Verification items for the finished model (mm, model axes). Give positions to 0.01 mm unless a question says otherwise; leave off trailing zeros. Order: outer loops, then holes, each group sorted by start corner. A loop starts at its lowest first (then second) coordinate and runs counter-clockwise, first axis right, second up.
(1) Gauge pin test, flat ends, axial feed: pin 1 (0.9 mm diameter, centred on y = 1.5, z = 267.5, fed in from -X); pin 2 (0.9 mm diameter, centred on x = 262, y = 1.5, fed in from -Z); pin 3 (1.5 mm diameter, centred on x = 227, y = 2, fed in from -Z); pin 4 (5 mm diameter, centred on x = 214, z = 124.5, fed in from +Y). Record the tip position at first contact, or that the pin passes through.
(2) Scan lines: L1, parallel to Z at x = 187, y = 2.8; L2, parallel to X at y = 2.4, z = 94.5; L3, parallel to X at y = 0.2, z = 154. Record each from-to range of solid material in increasing order.
(3) Sectioned sample at C-C on z = 191. Record the cut outline in (x, y).
(4) Sectioned sample at A-A on y = 1.3. Record the cut outline in (x, z).
(5) Sectioned sample at D-D on x = 137.5. Record the cut outline in (y, z).
(6) Sectioned sample at B-B on x = 178.5. Record the cut outline in (y, z), plus the area to 3 significant figures.
Autodesk Inventor part; units mm, degrees
ref_plane "YZ Plane" through (0, 0, 0) normal (1, 0, 0) x (0, 1, 0)
ref_plane "XZ Plane" through (0, 0, 0) normal (0, 1, 0) x (-1, 0, 0)
ref_plane "XY Plane" through (0, 0, 0) normal (0, 0, 1) x (1, 0, 0)
sketch "Sketch1" plane through (0, 0, 0) normal (0, 1, 0) x (-1, 0, 0)
  circle A0 centre (0, 0) radius 250
  circle A1 centre (0, 0) radius 270
  line L0 (270, 0) -> (250, 0)
  line L1 (-270, 0) -> (-250, 0)
  line L2 (0, 0) -> (-250, 0) construction
  line L3 (0, 250) -> (0, 0) construction
  line L4 (0, 270) -> (0, 250)
  line L5 (-250, 0) -> (-270, 0)
  line L6 (-254, 7) -> (-266, 7)
  line L7 (-266, 7) -> (-263.4522, 0)
  line L8 (-254, 7) -> (-256.5478, 0)
  line L9 (-260, 0) -> (-260, 7) construction
  line L10 (-255.1125, 57.8859) -> (-246.8075, 86.7134)
  line L11 (-246.8075, 86.7134) -> (-243.7326, 85.8275)
  line L12 (-243.7326, 85.8275) -> (-252.0376, 57)
  line L13 (-252.0376, 57) -> (-255.1125, 57.8859)
  line L14 (-255.1125, 57.8859) -> (-243.7326, 85.8275) construction
  line L15 (-246.8075, 86.7134) -> (-252.0376, 57) construction
  circle A2 centre (0, 0) radius 260 construction
  line L16 (-7, -254) -> (0, -256.5478)
  line L17 (-7, -266) -> (0, -263.4522)
  line L18 (-7, -254) -> (-7, -266)
  line L19 (254, -7) -> (256.5478, 0)
  line L20 (266, -7) -> (263.4522, 0)
  line L21 (254, -7) -> (266, -7)
  line L22 (7, 254) -> (0, 256.5478)
  line L23 (7, 266) -> (0, 263.4522)
  line L24 (7, 254) -> (7, 266)
  line L25 (-249.8769, -77.4256) -> (-257.0983, -48.3078)
  line L26 (-246.771, -76.6553) -> (-249.8769, -77.4256)
  line L27 (-253.9924, -47.5375) -> (-246.771, -76.6553)
  line L28 (-257.0983, -48.3078) -> (-253.9924, -47.5375)
  line L29 (-177.6869, -191.991) -> (-198.4998, -170.3849)
  line L30 (-175.3822, -189.771) -> (-177.6869, -191.991)
  line L31 (-196.1951, -168.1649) -> (-175.3822, -189.771)
  line L32 (-198.4998, -170.3849) -> (-196.1951, -168.1649)
  line L33 (-57.8859, -255.1125) -> (-86.7134, -246.8075)
  line L34 (-57, -252.0376) -> (-57.8859, -255.1125)
  line L35 (-85.8275, -243.7326) -> (-57, -252.0376)
  line L36 (-86.7134, -246.8075) -> (-85.8275, -243.7326)
  line L37 (77.4256, -249.8769) -> (48.3078, -257.0983)
  line L38 (76.6553, -246.771) -> (77.4256, -249.8769)
  line L39 (47.5375, -253.9924) -> (76.6553, -246.771)
  line L40 (48.3078, -257.0983) -> (47.5375, -253.9924)
  line L41 (191.991, -177.6869) -> (170.3849, -198.4998)
  line L42 (189.771, -175.3822) -> (191.991, -177.6869)
  line L43 (168.1649, -196.1951) -> (189.771, -175.3822)
  line L44 (170.3849, -198.4998) -> (168.1649, -196.1951)
  line L45 (255.1125, -57.8859) -> (246.8075, -86.7134)
  line L46 (252.0376, -57) -> (255.1125, -57.8859)
  line L47 (243.7326, -85.8275) -> (252.0376, -57)
  line L48 (246.8075, -86.7134) -> (243.7326, -85.8275)
  line L49 (249.8769, 77.4256) -> (257.0983, 48.3078)
  line L50 (246.771, 76.6553) -> (249.8769, 77.4256)
  line L51 (253.9924, 47.5375) -> (246.771, 76.6553)
  line L52 (257.0983, 48.3078) -> (253.9924, 47.5375)
  line L53 (177.6869, 191.991) -> (198.4998, 170.3849)
  line L54 (175.3822, 189.771) -> (177.6869, 191.991)
  line L55 (196.1951, 168.1649) -> (175.3822, 189.771)
  line L56 (198.4998, 170.3849) -> (196.1951, 168.1649)
  line L57 (57.8859, 255.1125) -> (86.7134, 246.8075)
  line L58 (57, 252.0376) -> (57.8859, 255.1125)
  line L59 (85.8275, 243.7326) -> (57, 252.0376)
  line L60 (86.7134, 246.8075) -> (85.8275, 243.7326)
  line L61 (-77.4256, 249.8769) -> (-48.3078, 257.0983)
  line L62 (-76.6553, 246.771) -> (-77.4256, 249.8769)
  line L63 (-47.5375, 253.9924) -> (-76.6553, 246.771)
  line L64 (-48.3078, 257.0983) -> (-47.5375, 253.9924)
  line L65 (-191.991, 177.6869) -> (-170.3849, 198.4998)
  line L66 (-189.771, 175.3822) -> (-191.991, 177.6869)
  line L67 (-168.1649, 196.1951) -> (-189.771, 175.3822)
  line L68 (-170.3849, 198.4998) -> (-168.1649, 196.1951)
  point P0 (260, 0)
  point P1 (-260, 0)
  point P2 (-249.4226, 71.8567)
  point P3 (-49.7078, 255.2041)
  point P4 (-253.5751, 57.4429)
  point P5 (-245.2701, 86.2705)
  point P6 (-7, -260)
  point P7 (260, -7)
  point P8 (7, 260)
  point P9 (-248.3239, -77.0405)
  point P10 (-255.5453, -47.9226)
  point P11 (-176.5346, -190.881)
  point P12 (-197.3475, -169.2749)
  point P13 (-57.4429, -253.5751)
  point P14 (-86.2705, -245.2701)
  point P15 (77.0405, -248.3239)
  point P16 (47.9226, -255.5453)
  point P17 (190.881, -176.5346)
  point P18 (169.2749, -197.3475)
  point P19 (253.5751, -57.4429)
  point P20 (245.2701, -86.2705)
  point P21 (248.3239, 77.0405)
  point P22 (255.5453, 47.9226)
  point P23 (176.5346, 190.881)
  point P24 (197.3475, 169.2749)
  point P25 (57.4429, 253.5751)
  point P26 (86.2705, 245.2701)
  point P27 (-77.0405, 248.3239)
  point P28 (-47.9226, 255.5453)
  point P29 (-190.881, 176.5346)
  point P30 (-169.2749, 197.3475)
  point P31 (-256.5478, 0)
  point P32 (0, 256.5478)
  point P33 (0, 263.4522)
  dimension "d0" = 500
  dimension "d1" = 540
  dimension "d4" = 90
  dimension "d5" = 7
  dimension "d6" = 70
  dimension "d8" = 12
  dimension "d13" = 3.2
  dimension "d14" = 30
  dimension "d15" = 50
  dimension "d20" = 520
  dimension "d23" = 360
  dimension "d27" = 360
extrude "Extrusion1" add sketch "Sketch1" along normal blind 3 contours A0 L1 L8 L6 L7 A1 L4 | L4 L23 L24 L22
properties part number "R50_CM_CIRCULO"
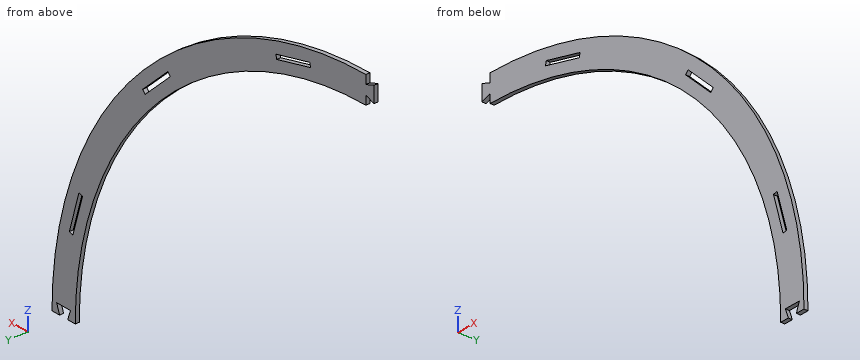
Ans:
1. pin 1: stops at x = 0
1. pin 2: stops at z = 7
1. pin 3: stops at z = 103.1
1. pin 4: stops at y = 3
2. L1: z = 165.92 to 178.05, 182.49 to 194.76
2. L2: x = 231.45 to 252.92
2. L3: x = 196.94 to 221.77
3. outline: (161.3, 0) - (173.56, 0) - (173.56, 3) - (161.3, 3) - close; (178.17, 0) - (190.84, 0) - (190.84, 3) - (178.17, 3) - close
4. outline: (-7, 254) - (0, 256.55) - (0, 250) arc R250 cw to (250, 0) - (256.55, 0) - (254, 7) - (266, 7) - (263.45, 0) - (270, 0) arc R270 ccw to (0, 270) - (0, 263.45) - (-7, 266) - close; hole (47.54, 253.99) - (76.66, 246.77) - (77.43, 249.88) - (48.31, 257.1) - close; hole (168.16, 196.2) - (189.77, 175.38) - (191.99, 177.69) - (170.38, 198.5) - close; hole (243.73, 85.83) - (252.04, 57) - (255.11, 57.89) - (246.81, 86.71) - close
5. outline: (0, 208.79) - (3, 208.79) - (3, 232.37) - (0, 232.37) - close
6. outline: (0, 175.04) - (3, 175.04) - (3, 186.24) - (0, 186.24) - close; (0, 190.68) - (3, 190.68) - (3, 202.58) - (0, 202.58) - close
6. area: 69.3 mm2
